```python
from build123d import *

# Parameters (mm, degrees)
F4_DEPTH = 25
F6_DEPTH = 40


with BuildPart() as f1:
    # F0 (on Top) → F1 (revolve)
    with BuildSketch(Plane.XY):
        Polygon((5, 53.16937), (0, 53.16937), (0, 0), (4, -1.83063), (4, -6.83063), (4, -21.83063), (8, -21.83063), (9, -20.83063), (9, 8.16937), (6, 8.16937), (6, 48.16937), (5, 48.16937), align=None)
    revolve(axis=Axis((0, 26.584685, 0), (0, -1, 0)))

    # F3 (on offset) → F4 (cut)
    with BuildSketch(Plane.XY.offset(7)):
        with BuildLine():
            ThreePointArc((-3, -13.83063), (0, -16.83063), (3, -13.83063))
            Line((3, -13.83063), (3, -7.83063))
            ThreePointArc((3, -7.83063), (0, -4.83063), (-3, -7.83063))
            Line((-3, -7.83063), (-3, -13.83063))
        make_face()
    extrude(amount=F4_DEPTH, mode=Mode.SUBTRACT)

    # F5 (on face) → F6 (join, through all)
    with BuildSketch(Plane(origin=(0, 48.16937, 0), x_dir=(-1, 0, 0), z_dir=(0, 1, 0))):
        with BuildLine():
            Line((0, 6), (-6, 6))
            Line((-6, 6), (-6, 0))
            ThreePointArc((-6, 0), (-4.242641, 4.242641), (0, 6))
        make_face()
        with BuildLine():
            ThreePointArc((0, -6), (-4.242641, -4.242641), (-6, 0))
            Line((-6, 0), (-6, -6))
            Line((-6, -6), (0, -6))
        make_face()
        with BuildLine():
            Line((6, -6), (6, 0))
            ThreePointArc((6, 0), (4.242641, -4.242641), (0, -6))
            Line((0, -6), (6, -6))
        make_face()
        with BuildLine():
            Line((6, 6), (0, 6))
            ThreePointArc((0, 6), (4.242641, 4.242641), (6, 0))
            Line((6, 0), (6, 6))
        make_face()
    extrude(amount=-F6_DEPTH)


solid = f1.part
```
The listing builds one solid part. Answer for the finished solid, in the listing's coordinates (mm). A direction names the side the tool comes from. Coordinates: 2 decimals unless noted, no trailing zeros. Write each loop counter-clockwise with the first axis right and the second up, starting at its lowest first coordinate (ties: lowest second). Pieces come first, ordered by that corner, then holes. Notation, with made-up numbers: (-34, -26.5) - (-2, -26.5) arc R22 ccw to (-2, 11.5) - close; hole circle Ø6 at (-25, -18.75). An arc over 180 degrees is marked (long way). Return JSON: item names as keys, results as strings. Group by question number.
Q1. The part is cut by section A-A on y = 21.5. Write down the section's boundary in (x, z).
Q2. Which of the six approach directions +Z, -Z, +X, -X, +Y, -Y give full straight-line access (tool end or side, diameter ignored) to faces 1 (the cylindrical face through (-0.867, -11.971, -3.905)), 2 (the flat face through (3, -11, 8)), 3 (the flat face through (0, 28, -6)), 4 (the cylindrical face through (-1.08, 50.7, -4.88)), 5 (the flat face through (6, 28, 0))?
Q3. For a pull along Y with two mould halves and no side action, classify faces 6 (the flat face through (0, 53.169, 0)), 7 (the flat face through (4, -21.831, -2)), 8 (the flat face through (-3, -11, 8)), 9 (the cylindrical face through (-0.07, -16.83, 7.76)) as +Y half, -Y half, draft (parallel to the pull), parting line (faces both ways), or undercut.
Q4. Find the intervals of material crossed by line 1 along Z through (x, y) = (0, -12.25); line 2 along Z through (x, y) = (3.75, 9), in increasing order. Write a range as [from, to].
Q5. Flat-ended cylindrical pins translate along their axes: pin 1 Ø6 at (y, z) = (-9, 6.5) entering from -X; pin 2 Ø3.5 at (y, z) = (37.5, 1) entering from +X; pin 3 Ø1.8 at (x, y) = (0, -11.5) entering from +Z; pin 4 Ø8 at (x, z) = (-2, -7) entering from +Y. Find the tip coordinate at first contact, or state that the pin passes through.
Evaluation:
{
 "1": {"outline": "(-6, -6) - (6, -6) - (6, 6) - (-6, 6) - close"},
 "2": {"face 1": "-Y", "face 2": "+Z", "face 3": "-Z, +X, -X, +Y", "face 4": "+Y", "face 5": "+Z, -Z, +X, +Y"},
 "3": {"face 6": "+Y half", "face 7": "-Y half", "face 8": "undercut", "face 9": "undercut"},
 "4": {"line 1": "z = [-9, -4], [4, 7]", "line 2": "z = [-6, 6]"},
 "5": {"pin 1": "stops at x = -8.29", "pin 2": "stops at x = 6", "pin 3": "stops at z = 7", "pin 4": "stops at y = 53.17"}
}
